from build123d import *

# Parameters (mm, degrees)
F0_W      = 254
F0_H      = 254
F1_DEPTH  = 508
F2_W      = 177.8
F2_H      = 177.8
F3_DEPTH  = 203.2
F5_DEPTH  = 127
F7_DEPTH  = 76.2
F9_DEPTH  = 254
F10_R     = 77.653267
F10_R_2   = 47.728315
F11_DEPTH = 127
F12_R     = 76.375648
F12_R_2   = 47.348432
F13_DEPTH = 152.4
F15_DEPTH = 203.2
F16_W     = 246.96593
F16_H     = 92.753515
F17_DEPTH = 152.4
F18_W     = 244.296044
F18_H     = 91.418564
F19_DEPTH = 152.4


with BuildPart() as f1:
    # F0 (on Front) → F1 (new body)
    with BuildSketch(Plane.XZ):
        with Locations((-4.823953, -9.921276)):
            Rectangle(F0_W, F0_H)
    extrude(amount=F1_DEPTH)

    # F2 (on Top) → F3 (join)
    with BuildSketch(Plane.XY):
        with Locations((-6.201372, -353.146609)):
            Rectangle(F2_W, F2_H)
    extrude(amount=F3_DEPTH)

    # F4 (on Top) → F5 (cut)
    with BuildSketch(Plane.XY):
        Polygon((-132.923797, -147.029117), (0, -12.960467), (0, 0), (-132.923797, 0), align=None)
        Polygon((0, 0), (0, -12.960467), (123.286948, -145.190179), (123.275883, 0), align=None)
    extrude(amount=F5_DEPTH, mode=Mode.SUBTRACT)

    # F6 (on Top) → F7 (cut)
    with BuildSketch(Plane.XY):
        Polygon((-132.923797, -145.192564), (-63.134633, 0), (-133.842081, 0), align=None)
        Polygon((61.751235, 0), (121.439323, -143.35601), (124.19416, 0), align=None)
    extrude(amount=-F7_DEPTH, mode=Mode.SUBTRACT)

    # F8 (on Top) → F9 (cut)
    with BuildSketch(Plane.XY):
        Polygon((121.439323, -452.815861), (-132.923797, -452.815861), (0, -520.768464), align=None)
    extrude(amount=-F9_DEPTH, mode=Mode.SUBTRACT)

    # F10 (on Right) → F11 (join)
    with BuildSketch(Plane.YZ):
        with Locations((-411.882162, -100.233831)):
            Circle(F10_R)
        with Locations((-80.955863, -128.580093)):
            Circle(F10_R_2)
    extrude(amount=F11_DEPTH)

    # F12 (on Right) → F13 (join)
    with BuildSketch(Plane.YZ):
        with Locations((-415.141463, -100.814395)):
            Circle(F12_R)
        with Locations((-80.068722, -127.513409)):
            Circle(F12_R_2)
    extrude(amount=-F13_DEPTH)

    # F14 (on Top) → F15 (cut)
    with BuildSketch(Plane.XY):
        Polygon((0, -440.878212), (-94.885923, -371.089071), (-94.885923, -442.663282), (82.948513, -442.663282), (82.948513, -364.321649), align=None)
    extrude(amount=F15_DEPTH, mode=Mode.SUBTRACT)

    # F16 (on Right) → F17 (cut)
    with BuildSketch(Plane.YZ):
        with Locations((-340.384193, 46.376757)):
            Rectangle(F16_W, F16_H)
    extrude(amount=-F17_DEPTH, mode=Mode.SUBTRACT)

    # F18 (on Right) → F19 (cut)
    with BuildSketch(Plane.YZ):
        with Locations((-339.716718, 45.709282)):
            Rectangle(F18_W, F18_H)
    extrude(amount=F19_DEPTH, mode=Mode.SUBTRACT)


solid = f1.part
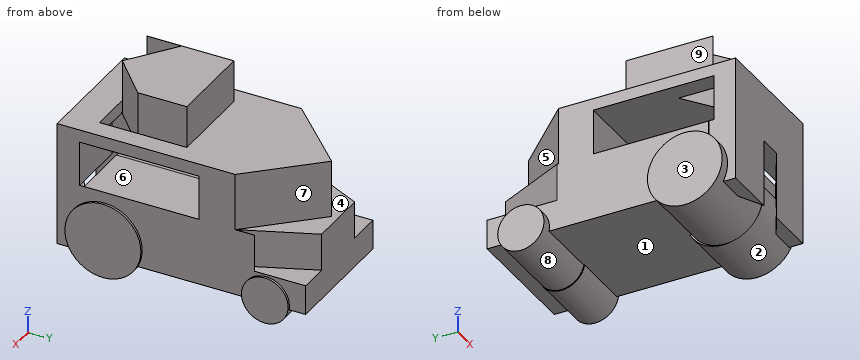
Verification items for the finished model (mm, model axes). Face numbers are marked on the shaded views. A direction names the side the tool comes from. Coordinates: 2 decimals unless noted, no trailing zeros. Loops run counter-clockwise (first coordinate to the right, second up) from the corner with the lowest first, then second, coordinate; pieces in that order, holes last. Notation, with made-up numbers: (67, 59.5) -> (89, 59.5) arc R27 ccw to (89, 96.5) -> close; hole circle Ø11 at (80, -39.5). An arc over 180 degrees is marked (long way). Answer as a JSON object with one key per item and string values. Group by question number.
Item 1: Sectioned sample at B-B on y = -247. Record the boundary of the cut face in (x, z), plus the area to 3 significant figures.
Item 2: Mould release check, pull along Z, two halves, no side actions. Record for the marked faces 1, 2, 3 and 4: +Z half, -Z half, draft (parallel to the pull), parting line (faces both ways), or undercut.
Item 3: Sectioned sample at D-D on x = -83.5. Record the boundary of the cut face in (y, z), plus the area to 3 significant figures.
Item 4: Scan lines: probe 1 along Z at (x, y) = (105.5, -255.5); probe 2 along Z at (x, y) = (-11, -247); probe 3 along X at (y, z) = (-325, 150.5). Record each from-to range of solid material in increasing order.
Item 5: Sectioned sample at C-C on x = -50. Record the boundary of the cut face in (y, z), plus the area to 3 significant figures.
Item 6: Depth check by flat-ended pin: pin 1 (21.5 mm diameter, centred on y = -422.5, z = 132, fed in from +X); pin 2 (5 mm diameter, centred on x = -109, y = -378.5, fed in from +Z); pin 3 (2 mm diameter, centred on x = 46, y = -242, fed in from -Z); pin 4 (10 mm diameter, centred on x = -43.5, z = 121.5, fed in from -Y). Enter the tip coordinate at first touch or a pass-through.
Item 7: Tool access check on the marked faces 5, 6, 7, 8 and 9. Record the directions out of +Z, -Z, +X, -X, +Y, -Y that give a thin tool (end or side, any length) a straight path to the whole face; none if there is none.
Item 8: Sectioned sample at A-A on z = 76.5. Record the boundary of the cut face in (x, y).
Evaluation:
{
 "1": {"outline": "(-131.82, -136.92) -> (122.18, -136.92) -> (122.18, 0) -> (-131.82, 0) -> close; (-131.82, 92.75) -> (0, 92.75) -> (0, 91.42) -> (122.18, 91.42) -> (122.18, 117.08) -> (-131.82, 117.08) -> close", "area": "41,100 mm²"},
 "2": {"face 1": "-Z half", "face 2": "undercut", "face 3": "draft", "face 4": "+Z half"},
 "3": {"outline": "(-508, -136.92) -> (-482.44, -136.92) arc R76.38 ccw to (-347.84, -136.92) -> (-126.47, -136.92) arc R47.35 ccw to (-33.66, -136.92) -> (0, -136.92) -> (0, -76.2) -> (-42.37, -76.2) -> (-42.37, 0) -> (-97.18, 0) -> (-97.18, 117.08) -> (-264.25, 117.08) -> (-264.25, 203.2) -> (-379.46, 203.2) -> (-379.46, 92.75) -> (-216.9, 92.75) -> (-216.9, 0) -> (-452.82, 0) -> (-452.82, -34.38) arc R76.38 ccw to (-478.08, -57.55) -> (-478.08, 0) -> (-463.87, 0) -> (-463.87, 92.75) -> (-442.66, 92.75) -> (-442.66, 117.08) -> (-508, 117.08) -> close", "area": "105,000 mm²"},
 "4": {"probe 1": "z = -136.92 to 0, 91.42 to 117.08", "probe 2": "z = -136.92 to 0, 92.75 to 117.08", "probe 3": "x = -95.1 to 82.7"},
 "5": {"outline": "(-508, -136.92) -> (-495.21, -136.92) -> (-495.21, 0) -> (-463.87, 0) -> (-463.87, 92.75) -> (-442.66, 92.75) -> (-442.66, 117.08) -> (-508, 117.08) -> close; (-452.82, -34.38) arc R76.38 ccw (long way) to (-347.84, -136.92) -> (-126.47, -136.92) arc R47.35 ccw to (-33.66, -136.92) -> (0, -136.92) -> (0, 0) -> (-63.39, 0) -> (-63.39, 117.08) -> (-264.25, 117.08) -> (-264.25, 203.2) -> (-404.1, 203.2) -> (-404.1, 92.75) -> (-216.9, 92.75) -> (-216.9, 0) -> (-452.82, 0) -> close", "area": "114,000 mm²"},
 "6": {"pin 1": "stops at x = 31.56", "pin 2": "stops at z = 117.08", "pin 3": "stops at z = -136.92", "pin 4": "stops at y = -508"},
 "7": {"face 5": "+Z, -X, +Y", "face 6": "+X, -X", "face 7": "+Z, +X, +Y", "face 8": "-X", "face 9": "+Z, -X, +Y, -Y"},
 "8": {"outline": "(-131.82, -508) -> (122.18, -508) -> (122.18, -461.86) -> (0, -461.86) -> (0, -463.87) -> (-131.82, -463.87) -> close; (-131.82, -216.9) -> (0, -216.9) -> (0, -217.57) -> (122.18, -217.57) -> (122.18, -144) -> (0, -12.96) -> (-131.82, -145.92) -> close"}
}
